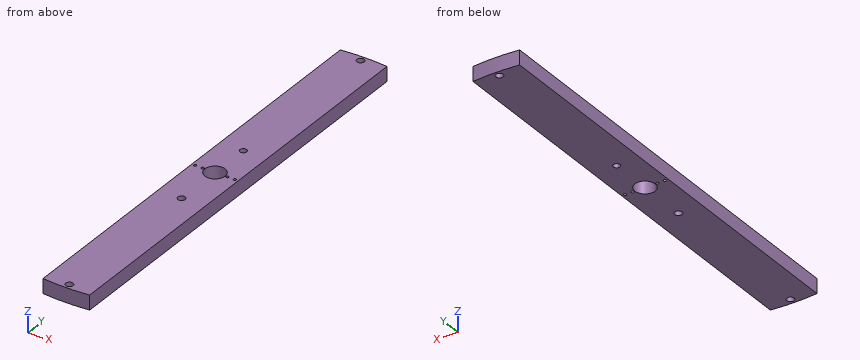
Autodesk Inventor part; units mm, degrees
ref_plane "YZ Plane" through (0, 0, 0) normal (1, 0, 0) x (0, 1, 0)
ref_plane "XZ Plane" through (0, 0, 0) normal (0, 1, 0) x (-1, 0, 0)
ref_plane "XY Plane" through (0, 0, 0) normal (0, 0, 1) x (1, 0, 0)
sketch "스케치1" plane through (0, 0, 0) normal (0, 0, 1) x (1, 0, 0)
  line L0 (-8, -75.5) -> (8, -75.5)
  line L1 (8, -75.5) -> (8, 75.5)
  line L2 (8, 75.5) -> (-8, 75.5)
  line L3 (-8, 75.5) -> (-8, -75.5)
  line L4 (-8, -75.5) -> (8, 75.5) construction
  line L5 (8, -75.5) -> (-8, 75.5) construction
  circle A0 centre (0, 0) radius 75.5
  circle A1 centre (0, 73.5) radius 1.25
  line L6 (0, 0) -> (8, 0) construction
  circle A2 centre (0, -73.5) radius 1.25
  circle A3 centre (0, 0) radius 3.5
  circle A4 centre (-4.25, 0) radius 0.5
  circle A5 centre (-6.85, 0) radius 0.5
  line L7 (0, 0) -> (0, 3.196) construction
  circle A6 centre (4.25, 0) radius 0.5
  circle A7 centre (6.85, 0) radius 0.5
  circle A8 centre (0, 14.3) radius 1.15
  circle A9 centre (0, -16.9) radius 1.25
  point P0 (0, 75.5)
  point P1 (8, -75.075)
  point P2 (8, 75.075)
  point P3 (-8, 75.075)
  point P4 (-8, -75.075)
  dimension "d1" = 151
  dimension "d0" = 16
  dimension "d2" = 2.5
  dimension "d3" = 73.5
  dimension "d4" = 7
  dimension "d5" = 1
  dimension "d6" = 1
  dimension "d7" = 8.5
  dimension "d8" = 12.7
  dimension "d9" = 2.3
  dimension "d13" = 14.3
  dimension "d14" = 2.5
  dimension "d15" = 16.9
extrude "돌출1" add sketch "스케치1" along normal blind 5 contours A0 L3 L1
properties part number "상단 서보모터 고정 판"
Source: CAD feature listing. Evaluate the final solid. Frame: model axes, mm. Coordinates: 2 decimals unless noted, no trailing zeros. Order: outer loops, then holes, each group sorted by start corner. A loop starts at its lowest first (then second) coordinate and runs counter-clockwise, first axis right, second up.
Item 1: Material intervals for line 1 (Y direction, x = 0, z = 2.25); line 2 (X direction, y = 73.5, z = 2.15); line 3 (Y direction, x = 0.5, z = 1.5), sorted ascending.
Output values:
line 1: y = -75.5 to -74.75, -72.25 to -18.15, -15.65 to -3.5, 3.5 to 13.15, 15.45 to 72.25, 74.75 to 75.5
line 2: x = -8 to -1.25, 1.25 to 8
line 3: y = -75.5 to -74.65, -72.35 to -18.05, -15.75 to -3.46, 3.46 to 13.26, 15.34 to 72.35, 74.65 to 75.5
Item 2: First-contact query: P1, Ø5.5, axis at x = 0, y = 0, coming from the +Z side; P2, Ø1.5, axis at x = -2.5, z = 3, coming from the -Y side. Flat tips, straight axial feed; report the tip coordinate or a pass-through.
Output values:
P1: passes through
P2: stops at y = -75.48
Item 3: Cut plane B-B (z = 2.4). Count the separate pieces of the cut face and the enclosed holes in it, plus the area to 3 significant figures.
Output values:
separate pieces: 1
enclosed holes: 9
area: 2,350 mm2
Item 4: Cut plane A-A (y = -16.9). Return loops of the section in (x, z).
Output values:
outline: (-8, 0) - (-1.25, 0) - (-1.25, 5) - (-8, 5) - close; (1.25, 0) - (8, 0) - (8, 5) - (1.25, 5) - close
